The listing builds one solid part. Answer for the finished solid, in the listing's coordinates (mm). A direction names the side the tool comes from. Coordinates: 2 decimals unless noted, no trailing zeros. Loops run counter-clockwise (first coordinate to the right, second up) from the corner with the lowest first, then second, coordinate; pieces in that order, holes last. Notation, with made-up numbers: (49.25, 73.5) - (100.25, 73.5) arc R21 ccw to (100.25, 86.5) - close; hole circle Ø2 at (28.5, 16.5). An arc over 180 degrees is marked (long way). Put each result on its own line as item: value.
```python
from build123d import *

# Parameters (mm, degrees)
SKETCH1_W           = 7
SKETCH1_H           = 30
BOSS_EXTRUDE1_DEPTH = 50
BOSS_EXTRUDE2_DEPTH = 6
BOSS_EXTRUDE3_DEPTH = 6
CUT_EXTRUDE1_DEPTH  = 75.779676383


with BuildPart() as part:
    # Sketch1 → Boss-Extrude1 (new body)
    with BuildSketch(Plane(origin=(0, 0, 0), x_dir=(1, 0, 0), z_dir=(0, 1, 0))):
        Polygon((-15, -15), (-15, 15), (-15, 22), (-22, 22), (-22, -15), align=None)
        Polygon((-15, 22), (-15, 15), (15, 15), (22, 15), (22, 22), align=None)
        with Locations((18.5, 0)):
            Rectangle(SKETCH1_W, SKETCH1_H)
    extrude(amount=BOSS_EXTRUDE1_DEPTH)

    # Sketch2 → Boss-Extrude2 (add)
    with BuildSketch(Plane(origin=(0, 0, -22), x_dir=(-1, 0, 0), z_dir=(0, 0, -1))):
        with BuildLine():
            Line((12.221813484, 35.179), (12.221813484, 0))
            Line((12.221813484, 0), (22, 0))
            Line((22, 0), (22, 50))
            Line((22, 50), (-22, 50))
            Line((-22, 50), (-22, 0))
            Line((-22, 0), (-15.078186516, 0))
            Line((-15.078186516, 0), (-15.078186516, 10.795))
            ThreePointArc((-15.078186516, 10.795), (-10.078186516, 15.795), (-5.078186516, 10.795))
            Line((-5.078186516, 10.795), (-5.078186516, 0))
            Line((-5.078186516, 0), (2.221813484, 0))
            Line((2.221813484, 0), (2.221813484, 35.179))
            ThreePointArc((2.221813484, 35.179), (7.221813484, 40.179), (12.221813484, 35.179))
        make_face()
    extrude(amount=BOSS_EXTRUDE2_DEPTH)

    # Sketch3 → Boss-Extrude3 (add)
    with BuildSketch(Plane(origin=(0, 0, -28), x_dir=(-1, 0, 0), z_dir=(0, 0, -1))):
        with BuildLine():
            Line((-7.078186516, 10.795), (-7.078186516, 0))
            Line((-7.078186516, 0), (4.221813484, 0))
            Line((4.221813484, 0), (4.221813484, 35.179))
            ThreePointArc((4.221813484, 35.179), (7.221813484, 38.179), (10.221813484, 35.179))
            Line((10.221813484, 35.179), (10.221813484, 0))
            Line((10.221813484, 0), (22, 0))
            Line((22, 0), (22, 50))
            Line((22, 50), (-22, 50))
            Line((-22, 50), (-22, 0))
            Line((-22, 0), (-13.078186516, 0))
            Line((-13.078186516, 0), (-13.078186516, 10.795))
            ThreePointArc((-13.078186516, 10.795), (-10.078186516, 13.795), (-7.078186516, 10.795))
        make_face()
    extrude(amount=BOSS_EXTRUDE3_DEPTH)

    # Sketch5 → Cut-Extrude1 (cut, through all)
    with BuildSketch(Plane.ZY.offset(22)):
        with BuildLine():
            ThreePointArc((0, 25), (1.171572875, 22.171572875), (4, 21))
            Line((4, 21), (4, 29))
            ThreePointArc((4, 29), (1.171572875, 27.828427125), (0, 25))
        make_face()
        with BuildLine():
            Line((4, 29), (4, 21))
            ThreePointArc((4, 21), (6.828427125, 22.171572875), (8, 25))
            ThreePointArc((8, 25), (6.828427125, 27.828427125), (4, 29))
        make_face()
    extrude(amount=-CUT_EXTRUDE1_DEPTH, mode=Mode.SUBTRACT)


solid = part.part
```
1) The part is cut by section A-A (z = -8.5). Give the vertices of the cut face in (x, y).
Found:
outline: (-22, 0) - (-15, 0) - (-15, 50) - (-22, 50) - close; (15, 0) - (22, 0) - (22, 50) - (15, 50) - close
2) For faces 5 (the face through (10, 8, -22)), 6 (the face through (-7.16, 38.18, -30.96)), 7 (the face through (-15, 25, -3)), determine the directions among +Z, -Z, +X, -X, +Y, -Y from which every point of the face is accessible in a straight line to the end or side of a thin tool.
Found:
face 5: -Y
face 6: -Z, -Y
face 7: +Z, +Y, -Y
3) The part is cut by section C-C (x = -18.5). Give the vertices of the cut face in (y, z).
Found:
outline: (0, -34) - (50, -34) - (50, 15) - (0, 15) - close; hole circle Ø8 at (25, 4)
4) Straight lines are drawn through the part: L1, parallel to X at y = 45.5, z = -7.5; L2, parallel to X at y = 15.5, z = -30; L3, parallel to X at y = 6, z = -23. For each, find the intervals that lie inside material, in ascending order. Write a range as [from, to].
Found:
L1: x = [-22, -15], [15, 22]
L2: x = [-22, -10.22], [-4.22, 22]
L3: x = [-22, -12.22], [-2.22, 5.08], [15.08, 22]
5) The part is cut by section B-B (y = 8.5). Give the vertices of the cut face in (x, z).
Found:
outline: (-22, -34) - (-10.22, -34) - (-10.22, -28) - (-12.22, -28) - (-12.22, -22) - (-2.22, -22) - (-2.22, -28) - (-4.22, -28) - (-4.22, -34) - (7.08, -34) - (7.08, -28) - (5.08, -28) - (5.08, -22) - (15.08, -22) - (15.08, -28) - (13.08, -28) - (13.08, -34) - (22, -34) - (22, 15) - (15, 15) - (15, -15) - (-15, -15) - (-15, 15) - (-22, 15) - close
6) Each of these flat-tipped pins is pushed along its axis until it touches: pin 1 (2 mm diameter, centred on x = -7.5, y = 24.5, fed in from +Z); pin 2 (3 mm diameter, centred on x = -6, y = 17.5, fed in from -Z). Where does it stop, or does it pass through?
Found:
pin 1: stops at z = -15
pin 2: stops at z = -22
7) For a pull along Z with two mould halves and no side action, classify faces 1 (the face through (-7.112, 40.178, -24.958)), 2 (the face through (0, 25, -34)), 3 (the face through (18, 25, 15)), 4 (the face through (15.078, 5, -25)) as pulls with the +Z half, pulls with the -Z half, needs draft (parallel to the pull), parting line crosses it, or undercut.
Found:
face 1: undercut
face 2: pulls with the -Z half
face 3: pulls with the +Z half
face 4: undercut
8) The part is cut by section D-D (z = 3). Give the vertices of the cut face in (x, y).
Found:
outline: (-22, 0) - (-15, 0) - (-15, 21.13) - (-22, 21.13) - close; (-22, 28.87) - (-15, 28.87) - (-15, 50) - (-22, 50) - close; (15, 0) - (22, 0) - (22, 21.13) - (15, 21.13) - close; (15, 28.87) - (22, 28.87) - (22, 50) - (15, 50) - close
